The listing builds one solid part. Answer for the finished solid, in the listing's coordinates (mm). A direction names the side the tool comes from. Give positions to 0.01 mm unless a question says otherwise; leave off trailing zeros. Write each loop counter-clockwise with the first axis right and the second up, starting at its lowest first coordinate (ties: lowest second). Pieces come first, ordered by that corner, then holes. Notation, with made-up numbers: (-27, -26.75) -> (10, -26.75) arc R24 ccw to (10, -9.75) -> close; hole circle Ø10 at (31.25, 4). An arc over 180 degrees is marked (long way). Put each result on its own line as item: value. Start each with the question number.
1) A cutting plane is placed at C-C (z = 0). Write down the section's boundary in (x, y).
2) A cutting plane is placed at B-B (x = 5). Write down the section's boundary in (y, z).
3) For faces 5 (the cylindrical face through (1.686, 9.824, 1.075)), 6 (the flat face through (-3.15, 6.5, -0.01)), 7 (the cylindrical face through (3, 6, 0)), determine the directions among +Z, -Z, +X, -X, +Y, -Y from which every point of the face is accessible in a straight line to the end or side of a thin tool.
4) A cutting plane is placed at A-A (y = 7). Write down the section's boundary in (x, z).
5) Flat-ended cylindrical pins translate along their axes: pin 1 Ø1.5 at (y, z) = (9, -2.5) entering from -X; pin 2 Ø1.5 at (y, z) = (8.5, -2) entering from +X; pin 3 Ø1.5 at (x, z) = (3.5, 2.5) entering from +Y. Find the tip coordinate at first contact, or state that the pin passes through.
6) Find the intervals of material crossed by line 1 along X through (y, z) = (7, -2.4); line 2 along Y through (x, z) = (0, 2.95); line 3 along Y through (x, z) = (3, 1.25), in increasing order. Write a range as from..to.
7) A cutting plane is placed at D-D (y = 11.25). Write down the section's boundary in (x, z), then the cut area to 3 significant figures.
8) For a pull along Y with two mould halves and no side action, classify faces 1 (the flat face through (-5, 4.5, 3)), 2 (the cylindrical face through (0, 5, -6)), 3 (the flat face through (-2, 15, -2)), 4 (the cylindrical face through (-3, 6, 0)) as released by +Y, released by -Y, zero draft, split by the parting line, or undercut.
from build123d import *

# Parameters (mm, degrees)
F2_SIZE  = 1
F3_R     = 1.5
F4_DEPTH = 25


with BuildPart() as f1:
    # F0 (on Right) → F1 (revolve)
    with BuildSketch(Plane.YZ):
        Polygon((4.5, 5.5), (0, 5.5), (0, 0), (4.5, 0), (4.5, 2), (15, 2), (15, 4.5), (6.5, 4.5), (6.5, 3), (5.5, 3), (5.5, 6), (4.5, 6), align=None)
    revolve(axis=Axis((0, 8.7408488616, 0), (0, 1, 0)))

    # F2
    f2_edges = [f1.edges().sort_by_distance(p)[0] for p in [
        (0, 15, -4.5),
        (0, 6.5, -4.5),
    ]]
    chamfer(f2_edges, length=F2_SIZE)

    # F3 (on Top) → F4 (cut, symmetric)
    with BuildSketch(Plane.XY):
        with Locations((0, 7)):
            Circle(F3_R)
    extrude(amount=F4_DEPTH, both=True, mode=Mode.SUBTRACT)


solid = f1.part
Reply:
1. outline: (-6, 4.5) -> (-5.5, 4.5) -> (-5.5, 0) -> (5.5, 0) -> (5.5, 4.5) -> (6, 4.5) -> (6, 5.5) -> (3, 5.5) -> (3, 6.5) -> (3.5, 6.5) -> (4.5, 7.5) -> (4.5, 14) -> (3.5, 15) -> (2, 15) -> (2, 4.5) -> (-2, 4.5) -> (-2, 15) -> (-3.5, 15) -> (-4.5, 14) -> (-4.5, 7.5) -> (-3.5, 6.5) -> (-3, 6.5) -> (-3, 5.5) -> (-6, 5.5) -> close
2. outline: (0, -2.29) -> (4.5, -2.29) -> (4.5, -3.32) -> (5.5, -3.32) -> (5.5, 3.32) -> (4.5, 3.32) -> (4.5, 2.29) -> (0, 2.29) -> close
3. face 5: +Y
3. face 6: -X
3. face 7: +X
4. outline: (-1.5, -3.71) -> (-1.5, -1.32) arc R2 cw to (-1.5, 1.32) -> (-1.5, 3.71) arc R4 ccw to start; (1.5, -3.71) arc R4 ccw to (1.5, 3.71) -> (1.5, 1.32) arc R2 cw to (1.5, -1.32) -> close
5. pin 1: stops at x = -4.15
5. pin 2: stops at x = 4.32
5. pin 3: stops at y = 14.95
6. line 1: x = -3.2..-1.5, 1.5..3.2
6. line 2: y = 0..5.5, 8.5..15
6. line 3: y = 0..5.5, 6.5..15
7. outline: circle Ø9 at (0, 0); hole circle Ø4 at (0, 0)
7. area: 51.1 mm2
8. face 1: released by -Y
8. face 2: zero draft
8. face 3: released by +Y
8. face 4: undercut
